from build123d import *

# Parameters (mm, degrees)
SKETCH1_W           = 25.4
SKETCH1_H           = 17.9
BOSS_EXTRUDE1_DEPTH = 4.9022
SKETCH2_R           = 2.5
BOSS_EXTRUDE2_DEPTH = 11.8618
SKETCH3_R           = 1.25
CUT_EXTRUDE1_DEPTH  = 17.764


with BuildPart() as part:
    # Sketch1 → Boss-Extrude1 (new body)
    with BuildSketch(Plane(origin=(0, 0, 0), x_dir=(1, 0, 0), z_dir=(0, 1, 0))):
        with Locations((-4.163944862, 2.526057393)):
            Rectangle(SKETCH1_W, SKETCH1_H)
    extrude(amount=BOSS_EXTRUDE1_DEPTH)

    # Sketch2 → Boss-Extrude2 (add)
    with BuildSketch(Plane.XZ):
        with Locations((-14.577944862, 3.687742607)):
            Circle(SKETCH2_R)
        with Locations((5.919855138, 3.687742607)):
            Circle(SKETCH2_R)
        with Locations((5.919855138, -9.190057393)):
            Circle(SKETCH2_R)
        with Locations((-14.577944862, -9.190057393)):
            Circle(SKETCH2_R)
    extrude(amount=BOSS_EXTRUDE2_DEPTH)

    # Sketch3 → Cut-Extrude1 (cut, through all)
    with BuildSketch(Plane.XZ.offset(11.8618)):
        with Locations((-14.577944862, 3.687742607)):
            Circle(SKETCH3_R)
        with Locations((-14.577944862, -9.190057393)):
            Circle(SKETCH3_R)
        with Locations((5.919855138, -9.190057393)):
            Circle(SKETCH3_R)
        with Locations((5.919855138, 3.687742607)):
            Circle(SKETCH3_R)
    extrude(amount=-CUT_EXTRUDE1_DEPTH, mode=Mode.SUBTRACT)


solid = part.part
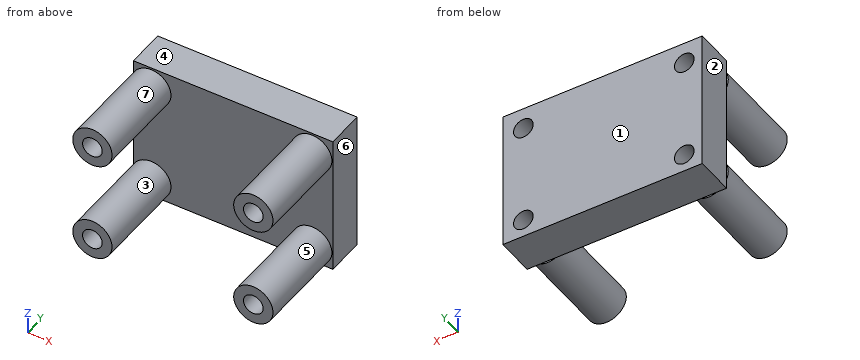
Verification items for the finished model (mm, model axes). Face numbers are marked on the shaded views. A direction names the side the tool comes from. Give positions to 0.01 mm unless a question says otherwise; leave off trailing zeros. Loops run counter-clockwise (first coordinate to the right, second up) from the corner with the lowest first, then second, coordinate; pieces in that order, holes last.
1) Sectioned sample at B-B, the plane y = 1. Enter the section's corners in (x, z), then the cut area to 3 significant figures.
2) Sectioned sample at C-C, the plane z = -7.5. Enter the section's corners in (x, y), then the cut area to 3 significant figures.
3) Sectioned sample at D-D, the plane x = -12.5. Enter the section's corners in (y, z), then the cut area to 3 significant figures.
4) Set-up check for the marked faces 1, 2 and 3: record each of +Z, -Z, +X, -X, +Y, -Y from which the full face is reachable in a straight line by a thin tool's end or side.
5) Depth check by flat-ended pin: pin 1 Ø8 at (y, z) = (-9, -5) entering from -X; pin 2 Ø3 at (x, z) = (-14.58, 3.69) entering from +Y; pin 3 Ø5.5 at (y, z) = (3, -2) entering from -X; pin 4 Ø4 at (x, z) = (-4.5, -8.5) entering from -Y. Enter the tip coordinate at first touch or a pass-through.
6) Thickness scan on line 1 along X through (y, z) = (-8.5, 3.75); line 2 along Z through (x, y) = (-15.25, 4); line 3 along Z through (x, y) = (5, -7). Record the ranges inside material, lowest first.
7) Sectioned sample at A-A, the plane y = -2. Enter the section's corners in (x, z).
8) Draft check along X on the marked faces 4, 5, 6 and 7. Enter one of: pulls with the +X half, pulls with the -X half, needs draft (parallel to the pull), parting line crosses it, or undercut.
Answers:
1. outline: (-16.86, -11.48) - (8.54, -11.48) - (8.54, 6.42) - (-16.86, 6.42) - close; hole circle Ø2.5 at (-14.58, -9.19); hole circle Ø2.5 at (-14.58, 3.69); hole circle Ø2.5 at (5.92, -9.19); hole circle Ø2.5 at (5.92, 3.69)
1. area: 435 mm2
2. outline: (-16.86, 0) - (-16.42, 0) - (-16.42, -11.86) - (-12.74, -11.86) - (-12.74, 0) - (4.08, 0) - (4.08, -11.86) - (7.76, -11.86) - (7.76, 0) - (8.54, 0) - (8.54, 4.9) - (-16.86, 4.9) - close
2. area: 212 mm2
3. outline: (-11.86, -10.58) - (0, -10.58) - (0, -11.48) - (4.9, -11.48) - (4.9, 6.42) - (0, 6.42) - (0, 5.08) - (-11.86, 5.08) - (-11.86, 2.3) - (0, 2.3) - (0, -7.8) - (-11.86, -7.8) - close
3. area: 154 mm2
4. face 1: +Z, -Z, +X, -X, +Y
4. face 2: +Z, -Z, -X, +Y
4. face 3: -Y
5. pin 1: stops at x = -17.07
5. pin 2: stops at y = 4.9
5. pin 3: stops at x = -16.86
5. pin 4: stops at y = 0
6. line 1: x = -17.08 to -15.83, -13.33 to -12.08, 3.42 to 4.67, 7.17 to 8.42
6. line 2: z = -11.48 to -10.24, -8.14 to 2.63, 4.74 to 6.42
6. line 3: z = -11.51 to -10.04, -8.34 to -6.87, 1.36 to 2.84, 4.53 to 6.01
7. outline: circle Ø5 at (-14.58, -9.19); circle Ø5 at (-14.58, 3.69); circle Ø5 at (5.92, -9.19); circle Ø5 at (5.92, 3.69); hole circle Ø2.5 at (-14.58, -9.19); hole circle Ø2.5 at (-14.58, 3.69); hole circle Ø2.5 at (5.92, -9.19); hole circle Ø2.5 at (5.92, 3.69)
8. face 4: needs draft
8. face 5: undercut
8. face 6: pulls with the +X half
8. face 7: undercut
